```python
from build123d import *

# Parameters (mm, degrees)
F1_DEPTH = 0.15
F2_DEPTH = 1.9
F3_W     = 0.15
F3_H     = 7
F4_DEPTH = 5
F6_DEPTH = 25
F7_R     = 0.5


# Not quite as in the source:
# - a feature names something its author has since deleted; it is built from what else it names


with BuildPart() as f1:
    # F0 (on Top) → F1 (new body)
    with BuildSketch(Plane.XY):
        with BuildLine():
            Line((10.1, -0.5), (10.1, -3.5))
            Line((10.1, -3.5), (20.2, -3.5))
            Line((20.2, -3.5), (30.3, -3.5))
            Line((30.3, -3.5), (30.3, -0.5))
            Line((30.3, -0.5), (25.7, -0.5))
            ThreePointArc((25.7, -0.5), (25.4171572875, -0.3828427125), (25.3, -0.1))
            Line((25.3, -0.1), (25.3, 0.1))
            ThreePointArc((25.3, 0.1), (25.4171572875, 0.3828427125), (25.7, 0.5))
            Line((25.7, 0.5), (30.3, 0.5))
            Line((30.3, 0.5), (30.3, 3.5))
            Line((30.3, 3.5), (20.2, 3.5))
            Line((20.2, 3.5), (10.1, 3.5))
            Line((10.1, 3.5), (10.1, 0.5))
            Line((10.1, 0.5), (14.7, 0.5))
            ThreePointArc((14.7, 0.5), (14.9828427125, 0.3828427125), (15.1, 0.1))
            Line((15.1, 0.1), (15.1, -0.1))
            ThreePointArc((15.1, -0.1), (14.9828427125, -0.3828427125), (14.7, -0.5))
            Line((14.7, -0.5), (10.1, -0.5))
        make_face()
        with BuildLine():
            Line((0, 3.5), (0, -3.5))
            Line((0, -3.5), (10.1, -3.5))
            Line((10.1, -3.5), (10.1, -0.5))
            Line((10.1, -0.5), (5.5, -0.5))
            ThreePointArc((5.5, -0.5), (5.2171572875, -0.3828427125), (5.1, -0.1))
            Line((5.1, -0.1), (5.1, 0.1))
            ThreePointArc((5.1, 0.1), (5.2171572875, 0.3828427125), (5.5, 0.5))
            Line((5.5, 0.5), (10.1, 0.5))
            Line((10.1, 0.5), (10.1, 3.5))
            Line((10.1, 3.5), (0, 3.5))
        make_face()
    extrude(amount=F1_DEPTH)

    # F2 (add): a face of the model
    f2_faces = [f1.faces().sort_by_distance(p)[0] for p in [
        (0, 0, 0.075),
    ]]
    extrude(f2_faces, amount=F2_DEPTH)

    # F3 (on face) → F4 (join)
    with BuildSketch(Plane(origin=(0, 0, 0), x_dir=(1, 0, 0), z_dir=(0, 0, -1))):
        with Locations((-1.825, 0)):
            Rectangle(F3_W, F3_H)
    extrude(amount=F4_DEPTH)

    # F5 (on face) → F6 (cut)
    with BuildSketch(Plane(origin=(-1.9, 0, 0), x_dir=(0, -1, 0), z_dir=(-1, 0, 0))):
        with BuildLine():
            ThreePointArc((0.5, -3.75), (0.3828427125, -3.4671572875), (0.1, -3.35))
            Line((0.1, -3.35), (-0.1, -3.35))
            ThreePointArc((-0.1, -3.35), (-0.3828427125, -3.4671572875), (-0.5, -3.75))
            Line((-0.5, -3.75), (-0.5, -5))
            Line((-0.5, -5), (0.5, -5))
            Line((0.5, -5), (0.5, -3.75))
        make_face()
    extrude(amount=-F6_DEPTH, mode=Mode.SUBTRACT)

    # F7
    f7_edges = [f1.edges().sort_by_distance(p)[0] for p in [
        (-1.9, 0, 0.15),
        (-1.75, 0, 0),
    ]]
    fillet(f7_edges, radius=F7_R)


solid = f1.part
```
Read the model definition and answer for the solid it produces. Units are mm, in the model's axes. Give positions to 0.01 mm unless a question says otherwise; leave off trailing zeros. Write each loop counter-clockwise with the first axis right and the second up, starting at its lowest first coordinate (ties: lowest second). Pieces come first, ordered by that corner, then holes. Notation, with made-up numbers: M 38.25,30 L 64.25,30 A14 cw 64.25,57 Z; hole C 65,41 d6. An arc over 180 degrees is marked long. Put each result on its own line as item: value. Start each with the question number.
1. The part is cut by section B-B, the plane y = -1.5. Give the vertices of the cut face in (x, z).
2. The part is cut by section C-C, the plane z = -2.65. Give the vertices of the cut face in (x, y), and give its area (3 significant figures).
3. Consider line 1 along Z through (x, y) = (5, -2); line 2 along X through (y, z) = (0.5, -0.25). Determine where each line is inside the solid, lowest interval first.
4. The part is cut by section D-D, the plane x = 2.5. Give the vertices of the cut face in (y, z), and give its area (3 significant figures).
5. The part is cut by section A-A, the plane x = 14. Give the vertices of the cut face in (y, z).
6. Each of these flat-tipped pins is pushed along its axis until it touches: pin 1 Ø4 at (x, y) = (26, 1) entering from -Z; pin 2 Ø1.5 at (x, z) = (8, -2) entering from -Y; pin 3 Ø1.3 at (y, z) = (0.5, -3.5) entering from +X. Where does it stop, or does it pass through?
Final values:
1. outline: M -1.9,-5 L -1.75,-5 L -1.75,-0.5 A0.5 cw -1.25,0 L 30.3,0 L 30.3,0.15 L -1.4,0.15 A0.5 ccw -1.9,-0.35 Z
2. outline: M -1.9,-3.5 L -1.75,-3.5 L -1.75,3.5 L -1.9,3.5 Z
2. area: 1.05 mm²
3. line 1: z = 0 to 0.15
3. line 2: x = -1.89 to -1.68
4. outline: M -3.5,0 L 3.5,0 L 3.5,0.15 L -3.5,0.15 Z
4. area: 1.05 mm²
5. outline: M -3.5,0 L -0.5,0 L -0.5,0.15 L -3.5,0.15 Z; M 0.5,0 L 3.5,0 L 3.5,0.15 L 0.5,0.15 Z
6. pin 1: stops at z = 0
6. pin 2: passes through
6. pin 3: stops at x = -1.75
